For this review, take the finished solid that the model builds, in its own axes (mm). Coordinates: 2 decimals unless noted, no trailing zeros. Write each loop counter-clockwise with the first axis right and the second up, starting at its lowest first coordinate (ties: lowest second). Pieces come first, ordered by that corner, then holes. Notation, with made-up numbers: (-32, 15) -> (-24, 15) arc R16 cw to (-24, 36) -> close; hole circle Ø9 at (62, -31). An arc over 180 degrees is marked (long way). Put each result on its own line as item: value. Start each with the question number.
Item 1: The part is to be moulded in two halves that separate along X. For faces 1 (the cylindrical face through (-68.87, 6.77, 1.52)), 2 (the cylindrical face through (88, -19, 3)), 3 (the cylindrical face through (-13.273, 12.082, 1.521)), 4 (the flat face through (-90, 0, 2)), say which applies: +X half, -X half, draft (parallel to the pull), parting line (faces both ways), or undercut.
Item 2: To check wall thickness, follow L1, parallel to Y at x = -13, z = 0.5; L2, parallel to X at y = 9, z = 1.95; L3, parallel to X at y = 8.5, z = 1.3. State the ranges of each line that lie inside material, in increasing order.
Item 3: Consider section A-A on x = 70. Give the boundary of the cut face in (y, z), and give its area (3 significant figures).
```python
from build123d import *

# Parameters (mm, degrees)
SZKIC1_W                    = 180
SZKIC1_H                    = 40
DODANIE_WYCI_GNI_CIE1_DEPTH = 5
ZAOKR_GLENIE1_R             = 5
SZKIC2_R                    = 2.1
WYTNIJ_WYCI_GNI_CIE1_DEPTH  = 5
SFAZOWANIE1_SIZE            = 2


with BuildPart() as part:
    # Szkic1 → Dodanie-wyciągnięcie1 (new body)
    with BuildSketch(Plane.XY):
        Rectangle(SZKIC1_W, SZKIC1_H)
    extrude(amount=DODANIE_WYCI_GNI_CIE1_DEPTH)

    # Zaokrąglenie1
    zaokr_glenie1_edges = [part.edges().sort_by_distance(p)[0] for p in [
        (90, -20, 2.5),
        (-90, -20, 2.5),
        (-90, 20, 2.5),
        (90, 20, 2.5),
    ]]
    fillet(zaokr_glenie1_edges, radius=ZAOKR_GLENIE1_R)

    # Szkic2 → Wytnij-wyciągnięcie1 (cut)
    with BuildSketch(Plane.XY.offset(5)):
        with Locations((-70, 5)):
            Circle(SZKIC2_R)
        with Locations((-13, 10)):
            Circle(SZKIC2_R)
        with Locations((13, 10)):
            Circle(SZKIC2_R)
        with Locations((70, 5)):
            Circle(SZKIC2_R)
    extrude(amount=-WYTNIJ_WYCI_GNI_CIE1_DEPTH, mode=Mode.SUBTRACT)

    # Sfazowanie1
    sfazowanie1_edges = [part.edges().sort_by_distance(p)[0] for p in [
        (-72.1, 5, 5),
        (-15.1, 10, 5),
        (10.9, 10, 5),
        (67.9, 5, 5),
    ]]
    chamfer(sfazowanie1_edges, length=SFAZOWANIE1_SIZE)


solid = part.part
```
Return value:
1. face 1: undercut
1. face 2: +X half
1. face 3: undercut
1. face 4: -X half
2. L1: -20 to 7.9, 12.1 to 20
2. L2: -90 to -14.85, -11.15 to 11.15, 14.85 to 90
2. L3: -90 to -14.47, -11.53 to 11.53, 14.47 to 90
3. outline: (-20, 0) -> (2.9, 0) -> (2.9, 3) -> (0.9, 5) -> (-20, 5) -> close; (7.1, 0) -> (20, 0) -> (20, 5) -> (9.1, 5) -> (7.1, 3) -> close
3. area: 175 mm^2
